Could you check a few things on this model? Use its own coordinates, in mm. A direction names the side the tool comes from. Round coordinates to 2 decimals unless told otherwise and drop trailing zeros. Write each loop counter-clockwise with the first axis right and the second up, starting at its lowest first coordinate (ties: lowest second). Pieces come first, ordered by that corner, then holes. Notation, with made-up numbers: (67, 5.5) - (107, 5.5) arc R31 cw to (107, 35.5) - close; hole circle Ø1 at (-8, -31). An arc over 180 degrees is marked (long way). Put each result on its own line as item: value.
from build123d import *
from OCP.BRepFilletAPI import BRepFilletAPI_MakeChamfer

# Parameters (mm, degrees)
SKETCH1_W           = 80
SKETCH1_H           = 50
BOSS_EXTRUDE1_DEPTH = 8
BOSS_EXTRUDE2_DEPTH = 80
SKETCH3_W           = 2.1
SKETCH3_H           = 35
BOSS_EXTRUDE3_DEPTH = 8.3
FILLET1_R           = 10
FILLET2_R           = 2
BOSS_EXTRUDE4_DEPTH = 10
CHAMFER2_SIZE       = 17.320508076
CHAMFER2_SIZE_2     = 10
SKETCH5_W           = 12.5
SKETCH5_H           = 9.237604307
BOSS_EXTRUDE5_DEPTH = 8.3
SKETCH6_W           = 6
SKETCH6_H           = 47.309401077
BOSS_EXTRUDE6_DEPTH = 2
CHAMFER3_SIZE       = 9
CHAMFER3_SIZE2      = 15.588457268
SKETCH7_W           = 17.5
SKETCH7_H           = 11.773502692
CUT_EXTRUDE1_DEPTH  = 12
SKETCH8_W           = 17.5
SKETCH8_H           = 15
CUT_EXTRUDE2_DEPTH  = 12
CUT_EXTRUDE3_DEPTH  = 12
CUT_EXTRUDE4_DEPTH  = 4


with BuildPart() as part:
    # Sketch1 → Boss-Extrude1 (new body)
    with BuildSketch(Plane(origin=(0, 0, 0), x_dir=(1, 0, 0), z_dir=(0, 1, 0))):
        Rectangle(SKETCH1_W, SKETCH1_H)
    extrude(amount=BOSS_EXTRUDE1_DEPTH)

    # Sketch2 → Boss-Extrude2 (add)
    with BuildSketch(Plane(origin=(40, 0, 0), x_dir=(0, 0, -1), z_dir=(1, 0, 0))):
        Polygon((15, 69.282032303), (11.535898385, 71.282032303), (-25, 8), (-20.381197846, 8), align=None)
    extrude(amount=-BOSS_EXTRUDE2_DEPTH)

    # Sketch3 → Boss-Extrude3 (add)
    with BuildSketch(Plane(origin=(0, 12.825317547, 22.214101615), x_dir=(1, 0, 0), z_dir=(0, 0.5000000000000041, 0.8660254037844364))):
        with Locations((-38.95, 15)):
            Rectangle(SKETCH3_W, SKETCH3_H)
        Polygon((-27.5, -5.57179677), (-27.5, -2.5), (-37.9, -2.5), (-40, -2.5), (-40, -5.57179677), align=None)
        Polygon((40, -5.57179677), (40, -2.5), (37.9, -2.5), (27.5, -2.5), (27.5, -5.57179677), align=None)
        with Locations((38.95, 15)):
            Rectangle(SKETCH3_W, SKETCH3_H)
    extrude(amount=BOSS_EXTRUDE3_DEPTH)

    # Fillet1
    fillet1_edges = [part.edges().sort_by_distance(p)[0] for p in [
        (-37.9, 12.735254038, 27.058107041),
        (37.9, 12.735254038, 27.058107041),
    ]]
    fillet(fillet1_edges, radius=FILLET1_R)

    # Fillet2
    fillet2_edges = [part.edges().sort_by_distance(p)[0] for p in [
        (-27.7, 10.660254038, 23.464101615),
        (-37.9, 30.145825623, 12.214101615),
        (27.7, 10.660254038, 23.464101615),
        (37.9, 30.145825623, 12.214101615),
        (34.971067812, 13.196783719, 21.999635521),
        (-34.971067812, 13.196783719, 21.999635521),
    ]]
    fillet(fillet2_edges, radius=FILLET2_R)

    # Sketch4 → Boss-Extrude4 (add)
    with BuildSketch(Plane.XY.offset(25)):
        Polygon((40, 0), (40, 8), (27.5, 8), (-27.5, 8), (-40, 8), (-40, 0), align=None)
    extrude(amount=BOSS_EXTRUDE4_DEPTH)

    # Chamfer2
    # the kernel refuses this chamfer: 17.320508076, 10 mm, written as the material it takes off along each edge
    with BuildSketch(Plane(origin=(-84.809639706, 8, 35), x_dir=(0, -0.999813220622208, 0.019326765612700497), z_dir=(1, 0, 0))) as chamfer2_piece_1:
        Polygon((CHAMFER2_SIZE * 0.999813220604, CHAMFER2_SIZE * 0.0193267656124), (-CHAMFER2_SIZE_2 * 0.0193267656127, CHAMFER2_SIZE_2 * 0.999813220622), (0, 0), align=None)
    extrude(amount=169.619279412, mode=Mode.SUBTRACT)

    # Sketch5 → Boss-Extrude5 (add)
    with BuildSketch(Plane(origin=(0, 12.825317547, 22.214101615), x_dir=(1, 0, 0), z_dir=(0, 0.49999999999999656, 0.8660254037844407))):
        with Locations((-33.75, -10.190598924)):
            Rectangle(SKETCH5_W, SKETCH5_H)
        with Locations((33.75, -10.190598924)):
            Rectangle(SKETCH5_W, SKETCH5_H)
    extrude(amount=BOSS_EXTRUDE5_DEPTH)

    # Sketch6 → Boss-Extrude6 (add)
    with BuildSketch(Plane(origin=(0, 16.975317547, 29.402112467), x_dir=(1, 0, 0), z_dir=(0, 0.5000000000000041, 0.8660254037844364))):
        with Locations((-37, 8.845299461)):
            Rectangle(SKETCH6_W, SKETCH6_H)
        with Locations((37, 8.845299461)):
            Rectangle(SKETCH6_W, SKETCH6_H)
    extrude(amount=BOSS_EXTRUDE6_DEPTH)

    # Chamfer3: one chamfer whose edges measure the first distance from different faces: ONE call of the kernel's chamfer builder (chamfer() names one face for all edges)
    chamfer3_edges_1 = [part.edges().sort_by_distance(p)[0] for p in [
        (-37, 5.15, 38.538863812),
    ]]
    chamfer3_side_1 = [part.faces().sort_by_distance(p)[0] for p in [
        (-34.086933045, 2.341954644, 33.675186585),
    ]]
    chamfer3_edges_2 = [part.edges().sort_by_distance(p)[0] for p in [
        (37, 5.15, 38.538863812),
    ]]
    chamfer3_side_2 = [part.faces().sort_by_distance(p)[0] for p in [
        (34.086933045, 2.341954644, 33.675186585),
    ]]
    chamfer3 = BRepFilletAPI_MakeChamfer(part.part.solid().wrapped)
    for e in chamfer3_edges_1:
        chamfer3.Add(CHAMFER3_SIZE, CHAMFER3_SIZE2, e.wrapped, chamfer3_side_1[0].wrapped)  # the first distance lies on this face
    for e in chamfer3_edges_2:
        chamfer3.Add(CHAMFER3_SIZE, CHAMFER3_SIZE2, e.wrapped, chamfer3_side_2[0].wrapped)  # the first distance lies on this face
    add(Compound.cast(chamfer3.Shape()), mode=Mode.REPLACE)

    # Sketch7 → Cut-Extrude1 (cut)
    with BuildSketch(Plane(origin=(0, 12.825317547, 22.214101615), x_dir=(1, 0, 0), z_dir=(0, 0.49999999999999656, 0.8660254037844407))):
        with Locations((18.75, -8.922649731)):
            Rectangle(SKETCH7_W, SKETCH7_H)
    extrude(amount=-CUT_EXTRUDE1_DEPTH, mode=Mode.SUBTRACT)

    # Sketch8 → Cut-Extrude2 (cut)
    with BuildSketch(Plane(origin=(0, 8, 0), x_dir=(1, 0, 0), z_dir=(0, 1, 0))):
        with Locations((18.75, -12.42820323)):
            Rectangle(SKETCH8_W, SKETCH8_H)
    extrude(amount=-CUT_EXTRUDE2_DEPTH, mode=Mode.SUBTRACT)

    # Sketch9 → Cut-Extrude3 (cut)
    with BuildSketch(Plane(origin=(0, 8, 0), x_dir=(1, 0, 0), z_dir=(0, 1, 0))):
        Polygon((-32, -12.381197846), (2, -12.381197846), (2, 3.07179677), (32, 3.07179677), (32, 17), (-32, 17), align=None)
    extrude(amount=-CUT_EXTRUDE3_DEPTH, mode=Mode.SUBTRACT)

    # Sketch10 → Cut-Extrude4 (cut)
    with BuildSketch(Plane(origin=(0, 12.825317547, 22.214101615), x_dir=(1, 0, 0), z_dir=(0, 0.500000000000004, 0.8660254037844365))):
        Polygon((-19.5, 7.5), (-19.5, 2.42820323), (2, 2.42820323), (2, 4.964101615), (19.5, 4.964101615), (19.5, 7.5), (27.9, 7.5), (27.9, 40.5), (32, 40.5), (32, 59.5), (-32, 59.5), (-32, 40.5), (-27.9, 40.5), (-27.9, 7.5), align=None)
    extrude(amount=-CUT_EXTRUDE4_DEPTH, mode=Mode.SUBTRACT)


solid = part.part
(1) If we mould it in two halves opening along Y, with no side actions, what happens to faces 1 (the face through (8.3, 8, -2.6)), 2 (the face through (32, 55, -4)), 3 (the face through (-37.04, 32.58, 22.7))? For each: pulls with the +Y half, pulls with the -Y half, needs draft (parallel to the pull), parting line crosses it, or undercut.
Values found:
face 1: undercut
face 2: needs draft
face 3: pulls with the +Y half
(2) I'm going to push flat-ended pins straight in: pin 1 (4 mm diameter, centred on y = 59.5, z = -3.5, fed in from +X); pin 2 (1 mm diameter, centred on x = -13, z = -7.5, fed in from +Y); pin 3 (1.5 mm diameter, centred on x = -10, z = 24, fed in from +Y); pin 4 (4 mm diameter, centred on x = -18.5, z = 20.5, fed in from +Y). Where does each tip first touch, or does it pass through?
Values found:
pin 1: stops at x = 40
pin 2: stops at y = 65.16
pin 3: stops at y = 11.03
pin 4: stops at y = 18.79
(3) Imagine slicing it at A-A, the plane x = -13.5. List the corners of the cut face in (y, z) for me.
Values found:
outline: (0, -25) - (8, -25) - (8, -17) - (0, -17) - close; (0, 12.38) - (8, 12.38) - (8, 20.38) - (12.93, 17.54) - (14.93, 21) - (0, 29.62) - close; (62.35, -11) - (69.28, -15) - (71.28, -11.54) - (64.35, -7.54) - close
(4) For faces 4 (the face through (19.5, 17, 17)), 5 (the face through (-34, 30, 23)), 6 (the face through (0.45, 63.37, -9.24)), 7 (the face through (-40, 23, 12)), 8 (the face through (19, 4, 4.928)), which set-ups out of +Z, -Z, +X, -X, +Y, -Y let a thin tool reach every point of the face, with its end or its side?
Values found:
face 4: -Z, +Y
face 5: +Z, +Y
face 6: +Z, -Y
face 7: +Z, -Z, -X, +Y, -Y
face 8: +Z, +Y, -Y
(5) Please list where these lines run through material, in increasing order: probe 1 along X at (y, z) = (56, -6.5); probe 2 along X at (y, z) = (21, 16.5); probe 3 along Y at (x, z) = (8, 8). Write a range as from..to.
Values found:
probe 1: x = -40..-32, 32..40
probe 2: x = -40..-27.9, 27.9..40
probe 3: y = 0..8
(6) Imagine slicing it at C-C, the plane y = 51. List the corners of the cut face in (x, z) for me.
Values found:
outline: (-40, -4.44) - (-32, -4.44) - (-32, 0.17) - (-40, 0.17) - close; (32, -4.44) - (40, -4.44) - (40, 0.17) - (32, 0.17) - close
(7) Imagine slicing it at B-B, the plane x = 21.5. List the corners of the cut face in (y, z) for me, then the cut area to 3 significant figures.
Values found:
outline: (0, -25) - (8, -25) - (8, -17) - (0, -17) - close; (0, -3.07) - (8, -3.07) - (8, 4.93) - (0, 4.93) - close; (8.2, 20.27) - (17.32, 15) - (19.32, 18.46) - (10.2, 23.73) - close; (62.35, -11) - (69.28, -15) - (71.28, -11.54) - (64.35, -7.54) - close
area: 202 mm^2
(8) Imagine slicing it at D-D, the plane z = 0.5. List the corners of the cut face in (x, y) for me, then the cut area to 3 significant figures.
Values found:
outline: (-40, 0) - (-32, 0) - (-32, 8) - (-40, 8) - close; (-40, 42.44) - (-27.9, 42.44) - (-27.9, 47.05) - (-32, 47.05) - (-32, 50.44) - (-40, 50.44) - close; (2, 0) - (40, 0) - (40, 8) - (2, 8) - close; (27.9, 42.44) - (40, 42.44) - (40, 50.44) - (32, 50.44) - (32, 47.05) - (27.9, 47.05) - close
area: 534 mm^2
